Could you check a few things on this model? Use its own coordinates, in mm. Face numbers are marked on the shaded views. A direction names the side the tool comes from. Round coordinates to 2 decimals unless told otherwise and drop trailing zeros. Loops run counter-clockwise (first coordinate to the right, second up) from the corner with the lowest first, then second, coordinate; pieces in that order, holes last. Notation, with made-up numbers: (7, 12) -> (13, 12) arc R14 ccw to (13, 30) -> close; hole circle Ø5 at (68.5, -17.5). An arc over 180 degrees is marked (long way). One line per item, written item: value.
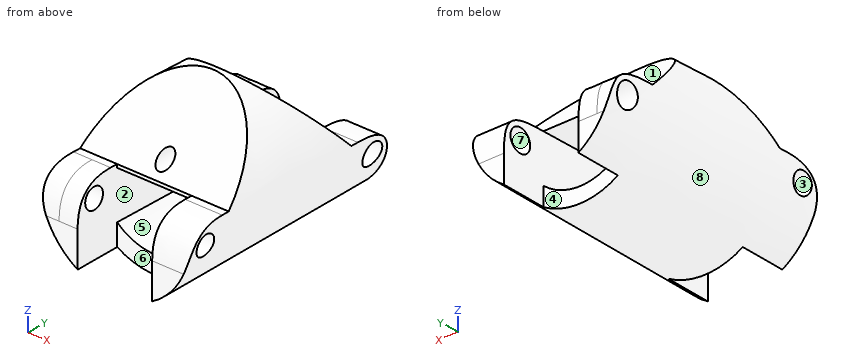
```python
from build123d import *

# Parameters (mm, degrees)
SKETCH1_R                     = 10
BOSS_EXTRUDE1_DEPTH           = 25
BOSS_EXTRUDE1_TAPER           = 1
BOSS_EXTRUDE1_OTHER_WAY_DEPTH = 6
BOSS_EXTRUDE1_OTHER_WAY_TAPER = -1
CUT_EXTRUDE1_DEPTH            = 29.796026679
CUT_EXTRUDE1_DEPTH_BACK       = 29.796026679
SKETCH3_W                     = 10
SKETCH3_H                     = 6
CUT_EXTRUDE2_DEPTH            = 25
CUT_EXTRUDE3_DEPTH            = 31.907255886
CUT_EXTRUDE3_DEPTH_BACK       = 31.907255886
SKETCH4_R                     = 1.5
FILLET2_SIZE                  = 5
CUT_EXTRUDE5_DEPTH            = 29.796026836
CUT_EXTRUDE5_DEPTH_BACK       = 29.796026836
SKETCH8_W                     = 10
SKETCH8_H                     = 6
CUT_EXTRUDE6_DEPTH            = 30.113855333
CUT_EXTRUDE7_DEPTH            = 29.75944341
CUT_EXTRUDE8_DEPTH            = 31.873174281
CUT_EXTRUDE8_DEPTH_BACK       = 31.873174281
SKETCH9_R                     = 1.351518808
FILLET3_SIZE                  = 5
SKETCH10_R                    = 1
CUT_EXTRUDE9_DEPTH            = 29.749923286


with BuildPart() as part:
    # Sketch1 → Boss-Extrude1 (new body)
    with BuildSketch(Plane(origin=(0, 0, 0), x_dir=(1, 0, 0), z_dir=(0, 1, 0))):
        Circle(SKETCH1_R)
    extrude(amount=BOSS_EXTRUDE1_DEPTH, taper=BOSS_EXTRUDE1_TAPER)

    # Sketch1 → Boss-Extrude1 other way (add)
    with BuildSketch(Plane(origin=(0, 0, 0), x_dir=(1, 0, 0), z_dir=(0, 1, 0))):
        Circle(SKETCH1_R)
    extrude(amount=-BOSS_EXTRUDE1_OTHER_WAY_DEPTH, taper=BOSS_EXTRUDE1_OTHER_WAY_TAPER)

    # Sketch2 → Cut-Extrude1 (cut, two sides: drawn at the far end of the back side and taken through both)
    with BuildSketch(Plane(origin=(0, 0, 0), x_dir=(0, 0, -1), z_dir=(1, 0, 0)).offset(-CUT_EXTRUDE1_DEPTH_BACK)):
        Polygon((-0.436376623, 25), (-0.436376623, 19), (-12.679815256, 6.756561367), (-12.679815256, 25), align=None)
    extrude(amount=CUT_EXTRUDE1_DEPTH + CUT_EXTRUDE1_DEPTH_BACK, mode=Mode.SUBTRACT)

    # Sketch3 → Cut-Extrude2 (cut)
    with BuildSketch(Plane.XY.offset(0.436376623)):
        with Locations((0, 22)):
            Rectangle(SKETCH3_W, SKETCH3_H)
    extrude(amount=-CUT_EXTRUDE2_DEPTH, mode=Mode.SUBTRACT)

    # Sketch4 → Cut-Extrude3 (cut, two sides: drawn at the far end of the back side and taken through both)
    with BuildSketch(Plane(origin=(-5, 0, 0), x_dir=(0, 0, -1), z_dir=(1, 0, 0)).offset(-CUT_EXTRUDE3_DEPTH_BACK)):
        with Locations(Location((2.063623377, 22.5, 0), (0, 0, 90))):
            Circle(SKETCH4_R)
    extrude(amount=CUT_EXTRUDE3_DEPTH + CUT_EXTRUDE3_DEPTH_BACK, mode=Mode.SUBTRACT)

    # Fillet2
    # a fillet whose section is not a circle: 5 mm, written as the material it takes off along each edge
    with BuildSketch(Plane(origin=(-7.5, 25, 0.436376623), x_dir=(0, -1, 0), z_dir=(1, 0, 0))) as fillet2_piece_1:
        with BuildLine():
            Bezier((FILLET2_SIZE, 0), (0, 0), (0, FILLET2_SIZE), weights=[1, 1.5, 1])
            Line((0, FILLET2_SIZE), (0, 0))
            Line((0, 0), (FILLET2_SIZE, 0))
        make_face()
    extrude(amount=29.553662519, mode=Mode.SUBTRACT)
    with BuildSketch(Plane(origin=(-22.053662519, 25, 0.436376623), x_dir=(0, 0, -1), z_dir=(1, 0, 0))) as fillet2_piece_2:
        with BuildLine():
            Bezier((FILLET2_SIZE, 0), (0, 0), (0, -FILLET2_SIZE), weights=[1, 1.5, 1])
            Line((0, -FILLET2_SIZE), (0, 0))
            Line((0, 0), (FILLET2_SIZE, 0))
        make_face()
    extrude(amount=29.553662519, mode=Mode.SUBTRACT)

    # Sketch7 → Cut-Extrude5 (cut, two sides: drawn at the far end of the back side and taken through both)
    with BuildSketch(Plane(origin=(0, 0, 0), x_dir=(0, 0, -1), z_dir=(1, 0, 0)).offset(-CUT_EXTRUDE5_DEPTH_BACK)):
        Polygon((-0.873019237, -6), (-0.873019237, 0), (-11.31781305, 10.444793812), (-11.31781305, -6), align=None)
    extrude(amount=CUT_EXTRUDE5_DEPTH + CUT_EXTRUDE5_DEPTH_BACK, mode=Mode.SUBTRACT)

    # Sketch8 → Cut-Extrude6 (cut, through all)
    with BuildSketch(Plane.XY.offset(0.873019237)):
        with Locations((0, -3)):
            Rectangle(SKETCH8_W, SKETCH8_H)
    extrude(amount=-CUT_EXTRUDE6_DEPTH, mode=Mode.SUBTRACT)

    # Sketch6 → Cut-Extrude7 (cut, through all)
    with BuildSketch(Plane(origin=(0, 19, 0), x_dir=(1, 0, 0), z_dir=(0, 1, 0))):
        with BuildLine():
            Line((5, 5.814090598), (5, -0.436376623))
            Line((5, -0.436376623), (-5, -0.436376623))
            Line((-5, -0.436376623), (-5, 5.814090598))
            ThreePointArc((-5, 5.814090598), (0, 7.668353766), (5, 5.814090598))
        make_face()
    extrude(amount=-CUT_EXTRUDE7_DEPTH, mode=Mode.SUBTRACT)

    # Sketch9 → Cut-Extrude8 (cut, two sides: drawn at the far end of the back side and taken through both)
    with BuildSketch(Plane(origin=(-5, 0, 0), x_dir=(0, 0, -1), z_dir=(1, 0, 0)).offset(-CUT_EXTRUDE8_DEPTH_BACK)):
        with Locations(Location((1.626980763, -3.5, 0), (0, 0, 90))):
            Circle(SKETCH9_R)
    extrude(amount=CUT_EXTRUDE8_DEPTH + CUT_EXTRUDE8_DEPTH_BACK, mode=Mode.SUBTRACT)

    # Fillet3
    # a fillet whose section is not a circle: 5 mm, written as the material it takes off along each edge
    with BuildSketch(Plane(origin=(22.566946591, -6, 0.873019237), x_dir=(0, 0, -1), z_dir=(-1, 0, 0))) as fillet3_piece_1:
        with BuildLine():
            Bezier((FILLET3_SIZE, 0), (0, 0), (0, -FILLET3_SIZE), weights=[1, 1, 1])
            Line((0, -FILLET3_SIZE), (0, 0))
            Line((0, 0), (FILLET3_SIZE, 0))
        make_face()
    extrude(amount=30.066946591, mode=Mode.SUBTRACT)
    with BuildSketch(Plane(origin=(7.5, -6, 0.873019237), x_dir=(0, 1, 0), z_dir=(-1, 0, 0))) as fillet3_piece_2:
        with BuildLine():
            Bezier((FILLET3_SIZE, 0), (0, 0), (0, FILLET3_SIZE), weights=[1, 1, 1])
            Line((0, FILLET3_SIZE), (0, 0))
            Line((0, 0), (FILLET3_SIZE, 0))
        make_face()
    extrude(amount=30.066946591, mode=Mode.SUBTRACT)

    # Sketch10 → Cut-Extrude9 (cut, through all)
    with BuildSketch(Plane(origin=(0, 19, 0), x_dir=(1, 0, 0), z_dir=(0, 1, 0))):
        with Locations(Location((0, -2.550318856, 0), (0, 0, 270))):
            Circle(SKETCH10_R)
    extrude(amount=-CUT_EXTRUDE9_DEPTH, mode=Mode.SUBTRACT)


solid = part.part
```
Item 1: I need wall thicknesses on line 1 (X direction, y = 16, z = -1.5); line 2 (Y direction, x = -8, z = -1.25); line 3 (Z direction, x = 2, y = 12). Which ranges of each line are inside material? Lowest first, please. Write a range as from..to.
Output:
line 1: x = -9.6..-5, 5..9.6
line 2: y = -5.39..-4.8, -2.2..21.24, 23.76..24.48
line 3: z = -9.58..-7.4, 0.44..7.44
Item 2: If we mould it in two halves opening along Y, with no side actions, what happens to the marked faces 1, 2 and 3? For each: released by +Y, released by -Y, zero draft, split by the parting line, or undercut.
Output:
face 1: released by +Y
face 2: zero draft
face 3: undercut
Item 3: For the marked faces 4, 5, 6, 7 and 8, which set-ups out of +Z, -Z, +X, -X, +Y, -Y let a thin tool reach every point of the face, with its end or its side?
Output:
face 4: +Z, -Z, +Y
face 5: +Y, -Y
face 6: +Z, -Z, -Y
face 7: +X, -X
face 8: +Y
Item 4: If we section it at B-B on y = -3.5: Count the separate pieces of the cut face and the enclosed holes in it, plus the area to 3 significant figures.
Output:
separate pieces: 4
enclosed holes: 0
area: 40.7 mm²
Item 5: If we section it at A-A on y = 8.5: List the corners of the cut face in (x, z) for me, plus the area to 3 significant figures.
Output:
outline: (-3.03, 9.37) arc R9.85 ccw (long way) to (3.03, 9.37) -> close; hole (-5, -5.81) arc R7.67 ccw to (5, -5.81) -> (5, 0.44) -> (-5, 0.44) -> close; hole circle Ø2 at (0, 2.55)
area: 225 mm²
Item 6: Will these pins go through, and if not, where does the flat tip stop? pin 1 Ø3 at (y, z) = (2, -5.5) entering from +X; pin 2 Ø1 at (x, y) = (-2, 6.5) entering from +Z; pin 3 Ø1 at (y, z) = (20, 1.5) entering from +X; pin 4 Ø0.5 at (x, y) = (7.5, -0.5) entering from +Z.
Output:
pin 1: stops at x = 9.13
pin 2: stops at z = 7.87
pin 3: passes through
pin 4: stops at z = 0.87
